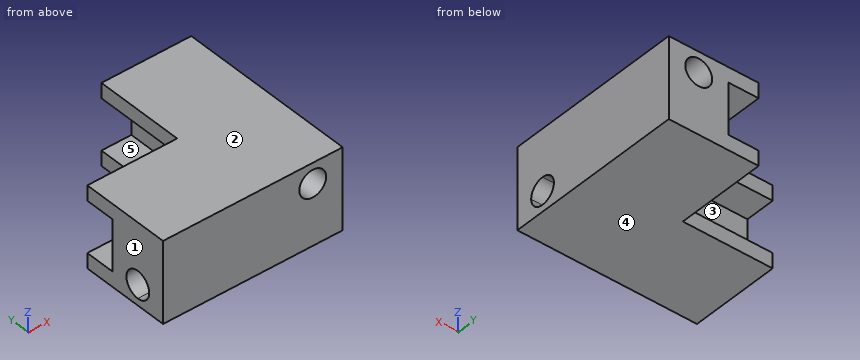
from build123d import *

# Parameters (mm, degrees)
F0_W      = 25
F0_H      = 10
F0_W_2    = 10
F0_H_2    = 30
F1_DEPTH  = 27
F3_DEPTH  = 5
F5_DEPTH  = 13.5
F7_DEPTH  = 10
F8_DEPTH  = 10
F9_R      = 4.5
F10_DEPTH = 60
F12_DEPTH = 60.001


with BuildPart() as f1:
    # F0 (on Top) → F1 (new body)
    with BuildSketch(Plane.XY):
        Polygon((20, 0), (10, 0), (10, -10), (-5, -10), (-5, -20), (20, -20), align=None)
        with Locations((-17.5, -15)):
            Rectangle(F0_W, F0_H)
        with Locations((15, 15)):
            Rectangle(F0_W_2, F0_H_2)
    extrude(amount=F1_DEPTH)

    # F0 (on Top) → F3 (join)
    with BuildSketch(Plane.XY):
        with Locations((5, 15)):
            Rectangle(F0_W_2, F0_H_2)
        Polygon((10, 0), (0, 0), (-30, 0), (-30, -10), (-5, -10), (10, -10), align=None)
    extrude(amount=F3_DEPTH)

    # F5 (cut, through all): a face of the model
    f5_faces = [f1.faces().sort_by_distance(p)[0] for p in [
        (-10, -10.7071067812, 27),
    ]]
    extrude(f5_faces, amount=-F5_DEPTH, mode=Mode.SUBTRACT)

    # F6: F1 across plane


with BuildPart() as f1_1:
    add(f1.part)
    add(f1.part.mirror(Plane(origin=(0, 0, 13.5), x_dir=(1, 0, 0), z_dir=(0, 0, -1))))

    # F7 (add): a face of the model
    f7_faces = [f1_1.faces().sort_by_distance(p)[0] for p in [
        (-5, -20, 13.5),
    ]]
    extrude(f7_faces, amount=F7_DEPTH)

    # F8 (add): a face of the model
    f8_faces = [f1_1.faces().sort_by_distance(p)[0] for p in [
        (20, 0, 13.5),
    ]]
    extrude(f8_faces, amount=F8_DEPTH)

    # F9 (on face) → F10 (cut, through all)
    with BuildSketch(Plane(origin=(0, 30, 0), x_dir=(-1, 0, 0), z_dir=(0, 1, 0))):
        with Locations((-20, 20.25)):
            Circle(F9_R)
    extrude(amount=-F10_DEPTH, mode=Mode.SUBTRACT)

    # F11 (on face) → F12 (cut, through all)
    with BuildSketch(Plane(origin=(-30, 0, 0), x_dir=(0, -1, 0), z_dir=(-1, 0, 0))):
        with BuildLine():
            ThreePointArc((24.5, 6.75), (23.1819805153, 9.9319805153), (20, 11.25))
            Line((20, 11.25), (20, 2.25))
            ThreePointArc((20, 2.25), (23.1819805153, 3.5680194847), (24.5, 6.75))
        make_face()
        with BuildLine():
            Line((20, 2.25), (20, 11.25))
            ThreePointArc((20, 11.25), (15.5, 6.75), (20, 2.25))
        make_face()
    extrude(amount=-F12_DEPTH, mode=Mode.SUBTRACT)


solid = f1_1.part
CAD build for the part. Positions are in the model's coordinates, mm. Face numbers are marked on the shaded views. A direction names the side the tool comes from. Round coordinates to 2 decimals unless told otherwise and drop trailing zeros. Write each loop counter-clockwise with the first axis right and the second up, starting at its lowest first coordinate (ties: lowest second). Pieces come first, ordered by that corner, then holes.
(1) Slice it at D-D, the plane y = 9. Write the cut outline in (x, z).
(2) Drop flat-ended pins along their axis: P1, Ø5, axis at y = 1, z = 15, coming from the -X side; P2, Ø5.5, axis at x = -11, z = 3.5, coming from the +Y side; P3, Ø4, axis at y = 20.5, z = 4.5, coming from the -X side. Give the stop position or say it passes through.
(3) Mould opens along Z. For the marked faces 1, 2 and 3 say: pulls with the +Z half, pulls with the -Z half, needs draft (parallel to the pull), parting line crosses it, or undercut.
(4) Probe line 1 along Z through (x, y) = (20, -13.5); line 2 along Y through (x, z) = (-26.5, 6.5); line 3 along Z through (x, y) = (-6, -6). List the from-to ranges inside material, lowest first.
(5) 3-axis set-ups, long thin cutter, end or side, ignore diameter. For the marked faces 4 and 5: which of +Z, -Z, +X, -X, +Y, -Y reach the whole face in a straight line?
(6) Slice it at B-B, the plane z = 20.25. Write the cut outline in (x, y).
(7) Slice it at A-A, the plane x = 20. Write the cut outline in (y, z), and give its area (3 significant figures).
(8) Slice it at C-C, the plane x = 5. Write the cut outline in (y, z).
From the geometry:
1. outline: (0, 0) - (30, 0) - (30, 27) - (0, 27) - (0, 22) - (10, 22) - (10, 5) - (0, 5) - close; hole circle Ø9 at (20, 20.25)
2. P1: stops at x = 10
2. P2: stops at y = 0
2. P3: stops at x = 0
3. face 1: needs draft
3. face 2: pulls with the +Z half
3. face 3: undercut
4. line 1: z = 0 to 15.75, 24.75 to 27
4. line 2: y = -30 to -24.49, -15.51 to -10
4. line 3: z = 0 to 5, 22 to 27
5. face 4: -Z, +X, -X, +Y, -Y
5. face 5: -X, +Y
6. outline: (-30, -30) - (15.5, -30) - (15.5, 30) - (10, 30) - (10, -10) - (-30, -10) - close; (24.5, -30) - (30, -30) - (30, 30) - (24.5, 30) - close
7. outline: (-30, 0) - (30, 0) - (30, 15.75) - (-30, 15.75) - close; (-30, 24.75) - (30, 24.75) - (30, 27) - (-30, 27) - close; hole circle Ø9 at (-20, 6.75)
7. area: 1,020 mm2
8. outline: (-30, 0) - (30, 0) - (30, 5) - (-10, 5) - (-10, 22) - (30, 22) - (30, 27) - (-30, 27) - close; hole circle Ø9 at (-20, 6.75)
